from build123d import *

# Parameters (mm, degrees)
STOCK_100996468_LAB1B_1_START         = 70
STOCK_100996468_LAB1B_1_OUTLINE_R     = 11
STOCK_100996468_LAB1B_1_DEPTH         = 170
STOCK_100996468_LAB1B_1_START_2       = 75
STOCK_100996468_LAB1B_1_2_OUTLINE_R   = 15
STOCK_100996468_LAB1B_1_2_OUTLINE_R_2 = 11
STOCK_100996468_LAB1B_1_2_DEPTH       = 5
FILLET1_R                             = 10


# Read off the part's stored shape, not the designer's step: Stock-100996468_Lab1B-1
with BuildPart() as part:
    # Stock-100996468_Lab1B-1 outline → Stock-100996468_Lab1B-1 (new body)
    with BuildSketch(Plane(origin=(0, 0, 0), x_dir=(1, 0, 0), z_dir=(0, 1, 0)).offset(STOCK_100996468_LAB1B_1_START)):
        with Locations((-62, 0)):
            Circle(STOCK_100996468_LAB1B_1_OUTLINE_R)
    extrude(amount=STOCK_100996468_LAB1B_1_DEPTH)

    # Stock-100996468_Lab1B-1 2 outline → Stock-100996468_Lab1B-1 2 (add)
    with BuildSketch(Plane(origin=(0, 0, 0), x_dir=(1, 0, 0), z_dir=(0, 1, 0)).offset(STOCK_100996468_LAB1B_1_START_2)):
        with Locations((-62, 0)):
            Circle(STOCK_100996468_LAB1B_1_2_OUTLINE_R)
        with Locations((-62, 0)):
            Circle(STOCK_100996468_LAB1B_1_2_OUTLINE_R_2, mode=Mode.SUBTRACT)
    extrude(amount=STOCK_100996468_LAB1B_1_2_DEPTH)

    # Fillet1
    fillet1_edges = [part.edges().sort_by_distance(p)[0] for p in [
        (-73, 240, 0),
    ]]
    fillet(fillet1_edges, radius=FILLET1_R)


solid = part.part
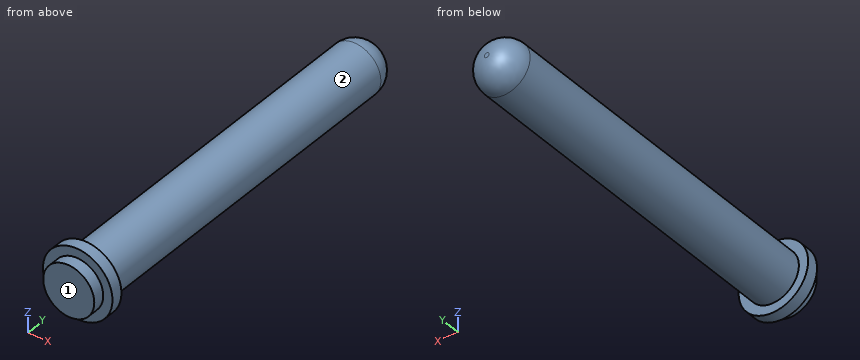
Check sheet for the modelled part. Datum: model origin and axes. Units: mm. Face numbers are marked on the shaded views. A direction names the side the tool comes from. Round coordinates to 2 decimals unless told otherwise and drop trailing zeros. Order: outer loops, then holes, each group sorted by start corner. A loop starts at its lowest first (then second) coordinate and runs counter-clockwise, first axis right, second up.
Q1. Set-up check for the marked faces 1 and 2: record each of +Z, -Z, +X, -X, +Y, -Y from which the full face is reachable in a straight line by a thin tool's end or side.
Filled sheet:
face 1: +Z, -Z, +X, -X, -Y
face 2: +Y
Q2. Depth check by flat-ended pin: P1, Ø1, axis at y = 189, z = 4, coming from the +X side; P2, Ø3, axis at y = 136.5, z = 0.5, coming from the -X side; P3, Ø4, axis at x = -57.5, y = 220.5, coming from the +Z side. Enter the tip coordinate at first touch or a pass-through.
Filled sheet:
P1: stops at x = -51.57
P2: stops at x = -73
P3: stops at z = 10.71
Q3. Scan lines: L1, parallel to Y at x = -64, z = -11; L2, parallel to X at y = 94.5, z = -5.75; L3, parallel to X at y = 198, z = -6.25. Record each from-to range of solid material in increasing order.
Filled sheet:
L1: y = 75 to 80
L2: x = -71.38 to -52.62
L3: x = -71.05 to -52.95
Q4. Cross-section at A-A, the plane y = 168. Enter the section's corners in (x, z).
Filled sheet:
outline: circle Ø22 at (-62, 0)
